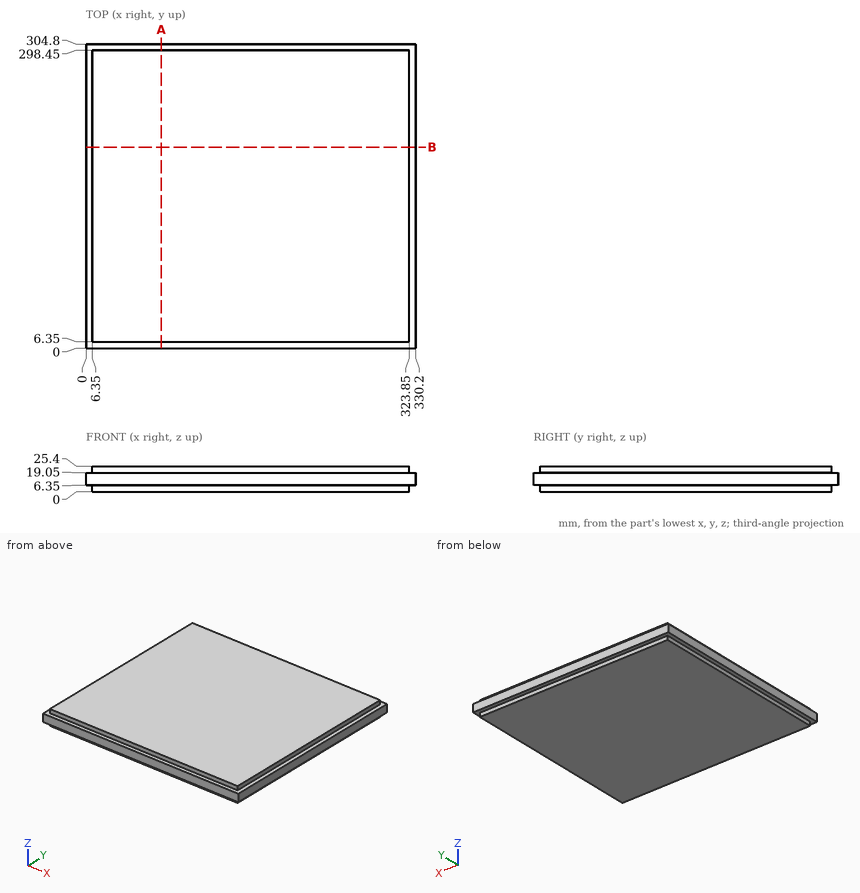
Design review of the part shown in the three views and the two pictorial views. Dimensions are in mm from the part's minimum x, y and z. Give positions to 0.01 mm unless a question says otherwise; leave off trailing zeros. Write each loop counter-clockwise with the first axis right and the second up, starting at its lowest first coordinate (ties: lowest second). Pieces come first, ordered by that corner, then holes. Notation, with made-up numbers: M 46,60.25 L 72,60.25 A25 cw 72,77.25 Z; hole C -30,32.5 d10. An arc over 180 degrees is marked long. One line per item, written item: value.
1) Take a section at B-B, the plane y = 201.5. Write out the cut boundary in (x, z), then the cut area to 3 significant figures.
Results are:
outline: M 0,6.35 L 6.35,6.35 L 6.35,0 L 323.85,0 L 323.85,6.35 L 330.2,6.35 L 330.2,19.05 L 323.85,19.05 L 323.85,25.4 L 6.35,25.4 L 6.35,19.05 L 0,19.05 Z
area: 8,230 mm²
2) For P1, Ø7, axis at y = 97.5, z = 23.5, coming from the +X side; P2, Ø1, axis at x = 68.5, y = 245.5, coming from the -Z side; P3, Ø1.9, axis at x = 165.5, z = 23.5, coming from the -Y side; P4, Ø5, axis at x = 138, z = 3, coming from the +Y side, all flat-tipped, find the tip position at first contact; note any pin that passes through.
Results are:
P1: stops at x = 323.85
P2: stops at z = 0
P3: stops at y = 6.35
P4: stops at y = 298.45
3) Take a section at A-A, the plane x = 75.5. Write out the cut boundary in (y, z), then the cut area to 3 significant figures.
Results are:
outline: M 0,6.35 L 6.35,6.35 L 6.35,0 L 298.45,0 L 298.45,6.35 L 304.8,6.35 L 304.8,19.05 L 298.45,19.05 L 298.45,25.4 L 6.35,25.4 L 6.35,19.05 L 0,19.05 Z
area: 7,580 mm²
4) For line 1 (Y direction, x = 136, z = 3); line 2 (X direction, y = 180.5, z = 6), list the stretches that pass through material, from the lowest coordinate up. Write a range as from..to.
Results are:
line 1: y = 6.35..298.45
line 2: x = 6.35..323.85
